Design review of the part built by this model. Coordinates are the model's own, in mm. Coordinates: 2 decimals unless noted, no trailing zeros.
from build123d import *

# Parameters (mm, degrees)
F1_ANGLE = 180
F2_W     = 27.4360350213
F2_H     = 1.27
F8_DEPTH = 38.1


# Not quite as in the source:
# - the program builds the solid bodies; features that only make, move or delete a surface that nothing else refers to are left out


with BuildPart() as f1:
    # F0 (on Top) → F1 (revolve)
    with BuildSketch(Plane.XY):
        with BuildLine():
            Line((32.5160350213, 0), (-36.8259649787, 0))
            ThreePointArc((-36.8259649787, 0), (-2.1549649787, -35.0073002846), (32.5160350213, 0))
        make_face()
    revolve(axis=Axis((-2.1549649787, 0, 0), (-1, 0, 0)), revolution_arc=F1_ANGLE)

    # F2 (on Front) → F3 (revolve)
    with BuildSketch(Plane.XZ):
        with Locations((13.7180175106, -0.635)):
            Rectangle(F2_W, F2_H)
    revolve(axis=Axis((0, 0, -0.635), (0, 0, -1)))

    # F4: F1 across face


with BuildPart() as f1_1:
    add(f1.part)
    add(f1.part.mirror(Plane(origin=(0, 0, -1.27), x_dir=(1, 0, 0), z_dir=(0, 0, -1))))

    # F7 (on Right) → F8 (join)
    with BuildSketch(Plane.YZ):
        with BuildLine():
            ThreePointArc((-0.7505157715, 4.4294735411), (-4.7934462503, -8.0205740429), (7.1645930807, -2.6957015507))
            ThreePointArc((7.1645930807, -2.6957015507), (4.7934462503, 2.6291709415), (-0.7505157715, 4.4294735411))
        make_face()
    extrude(amount=-F8_DEPTH)


solid = f1_1.part
Q1. Clearance check with flat-ended pins moving along their axes: pin 1 Ø20.5 at (x, y) = (-4.5, -11.5) entering from -Z; pin 2 Ø1.5 at (y, z) = (23.5, -8.5) entering from -X; pin 3 Ø4 at (x, z) = (5, -29) entering from -Y. State where each tip first meets the part, or that it passes through.
Q2. The part is to be moulded in two halves that separate along Z. For faces 1 (the flat face through (-25, -13, 0)), 2 (the flat face through (-38.1, 0, -3)), say which applies: pulls with the +Z half, pulls with the -Z half, needs draft (parallel to the pull), parting line crosses it, or undercut.
Q3. For line 1 (Y direction, x = 16.5, z = 11); line 2 (X direction, y = 17.5, z = 1); line 3 (Z direction, x = 25, y = 3), list the stretches that pass through material, from the lowest coordinate up.
Entries:
1. pin 1: stops at z = -37.52
1. pin 2: stops at x = -27.96
1. pin 3: stops at y = -24.07
2. face 1: undercut
2. face 2: needs draft
3. line 1: y = -27.44 to 27.44
3. line 2: x = -32.26 to 27.95
3. line 3: z = -24.23 to 21.69
